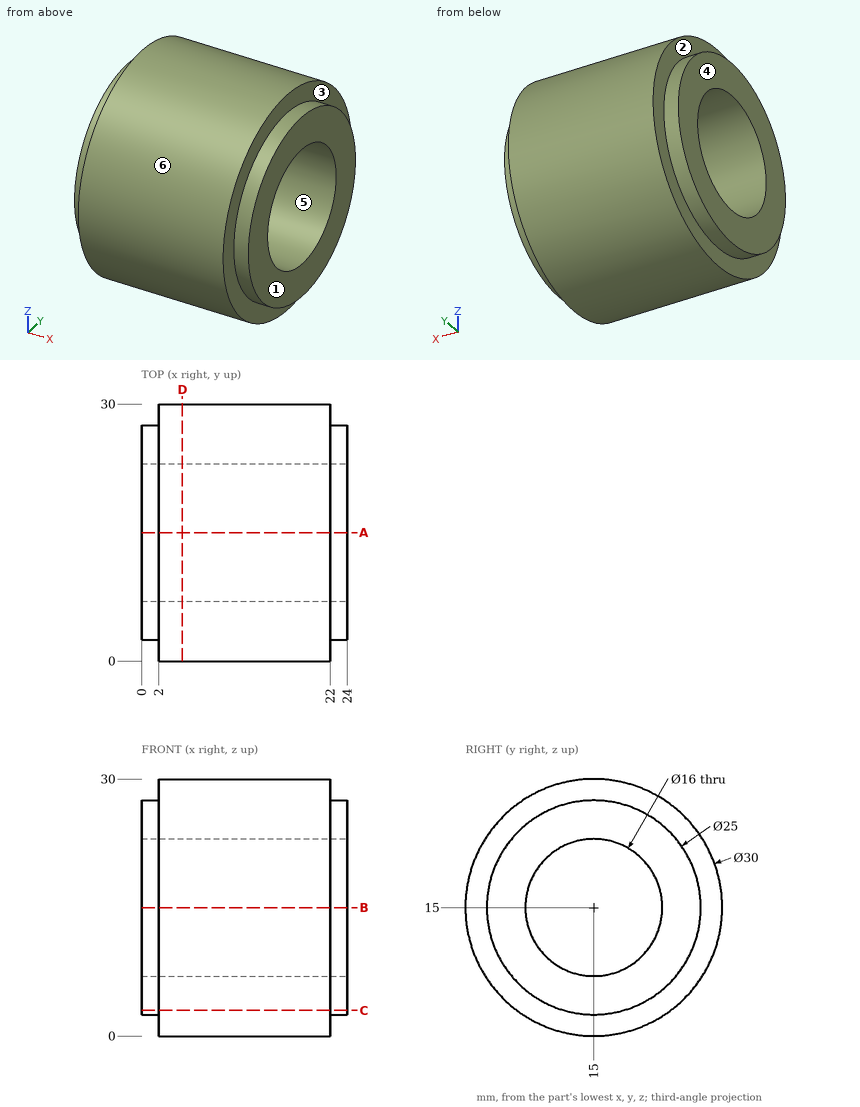
Study the drawing (mm; zero at the part's minimum x, y, z) and answer. A direction names the side the tool comes from. Round coordinates to 2 decimals unless told otherwise and drop trailing zeros. Write each loop counter-clockwise with the first axis right and the second up, starting at its lowest first coordinate (ties: lowest second). Pieces come first, ordered by that corner, then holes. Notation, with made-up numbers: (40, 58) - (65, 58) arc R26 cw to (65, 88) - close; hole circle Ø8 at (33, -27.75). An arc over 180 degrees is marked (long way). Use a Markdown table: item, result. Add a question column.
1. The part is cut by section D-D (x = 4.75). Write down the section's boundary in (y, z).
2. The part is cut by section A-A (y = 15). Write down the section's boundary in (x, z), and give its area (3 significant figures).
3. Flat-ended cylindrical pins translate along their axes: P1, Ø4, axis at x = 2.5, z = 10.5, coming from the -Y side; P2, Ø6, axis at x = 4, y = 16, coming from the -Z side; P3, Ø2, axis at x = 21.5, z = 27, coming from the +Y side; P4, Ø4, axis at x = 12.5, y = 7.5, coming from the -Z side. Find the tip coordinate at first contact, or state that the pin passes through.
4. The part is cut by section C-C (z = 3). Write down the section's boundary in (x, y).
5. A tool of negligible diameter and unlimited length cuts with its end or side. For the marked faces 1, 2 and 3, from which of +Z, -Z, +X, -X, +Y, -Y can it reach the whole face along a straight path? Write none if from no direction.
6. For a pull along Y with two mould halves and no side action, classify the marked faces 4, 5 and 6 as +Y half, -Y half, draft (parallel to the pull), parting line (faces both ways), or undercut.
7. Consider line 1 (Y direction, x = 16, z = 10.75); line 2 (Z direction, x = 8.25, y = 17.25); line 3 (Y direction, x = 4.75, z = 16.5). Determine where each line is inside the solid, lowest interval first.
Reported:
| question | item | result |
|---|---|---|
| 1 | outline | circle Ø30 at (15, 15); hole circle Ø16 at (15, 15) |
| 2 | outline | (0, 2.5) - (2, 2.5) - (2, 0) - (22, 0) - (22, 2.5) - (24, 2.5) - (24, 7) - (0, 7) - close; (0, 23) - (24, 23) - (24, 27.5) - (22, 27.5) - (22, 30) - (2, 30) - (2, 27.5) - (0, 27.5) - close |
| 2 | area | 316 mm^2 |
| 3 | P1 | y = 0.21 |
| 3 | P2 | z = 0 |
| 3 | P3 | y = 25.2 |
| 3 | P4 | z = 1.04 |
| 4 | outline | (0, 11.5) - (2, 11.5) - (2, 6) - (22, 6) - (22, 11.5) - (24, 11.5) - (24, 18.5) - (22, 18.5) - (22, 24) - (2, 24) - (2, 18.5) - (0, 18.5) - close |
| 5 | face 1 | +Z, -Z, +X, +Y, -Y |
| 5 | face 2 | -X |
| 5 | face 3 | +X |
| 6 | face 4 | draft |
| 6 | face 5 | undercut |
| 6 | face 6 | parting line |
| 7 | line 1 | 0.61 to 8.22, 21.78 to 29.39 |
| 7 | line 2 | 0.17 to 7.32, 22.68 to 29.83 |
| 7 | line 3 | 0.08 to 7.14, 22.86 to 29.92 |
